For this review, take the finished solid that the model builds, in its own axes (mm). Face numbers are marked on the shaded views. Round coordinates to 2 decimals unless told otherwise and drop trailing zeros. Write each loop counter-clockwise with the first axis right and the second up, starting at its lowest first coordinate (ties: lowest second). Pieces come first, ordered by that corner, then holes. Notation, with made-up numbers: (76.25, 85.25) -> (128.25, 85.25) arc R14 cw to (128.25, 91.25) -> close; hole circle Ø3 at (-21, 77). An arc over 180 degrees is marked (long way). Answer in a Markdown table with one row per item.
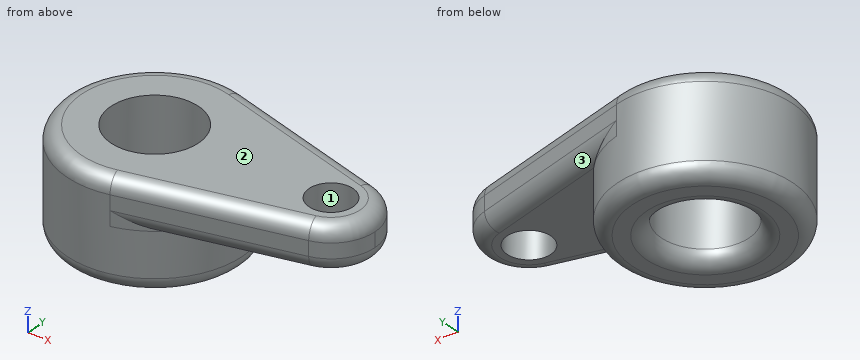
from build123d import *
from build123d import SkipClean  # not in build123d's __all__

# Parameters (mm, degrees)
F0_R         = 15
F0_R_2       = 7.5
F1_DEPTH     = 15
F2_DEPTH     = 20
F3_R         = 5
F4_T1_DEPTH  = 58.0947501931
F4_T3_DEPTH  = 58.0947501931
F4_T8_DEPTH  = 79.3447501931
F4_S9_R      = 30
F4_T10_DEPTH = 43
F4_T12_ANGLE = 151.0449756281
F4_T14_ANGLE = 151.0449756281
F4_T18_DEPTH = 79.3447501931
F4_S19_R     = 30
F4_T20_DEPTH = 43
F4_T22_ANGLE = 208.9550243719


# Not quite as in the source:
# - a fillet or chamfer that OpenCascade refuses, or shapes differently, is made with other operations: its cross-section is extruded or revolved along the edge and cut away or added


with BuildPart() as f1:
    # F0 (on Top) → F1 (new body)
    with BuildSketch(Plane.XY):
        with BuildLine():
            ThreePointArc((7.5, -29.0473750966), (23.7170824513, -18.3711730709), (30, 0))
            ThreePointArc((30, 0), (23.7170824513, 18.3711730709), (7.5, 29.0473750966))
            ThreePointArc((7.5, 29.0473750966), (-30, 0), (7.5, -29.0473750966))
        make_face()
        Circle(F0_R, mode=Mode.SUBTRACT)
        with BuildLine():
            ThreePointArc((7.5, 29.0473750966), (23.7170824513, 18.3711730709), (30, 0))
            ThreePointArc((30, 0), (23.7170824513, -18.3711730709), (7.5, -29.0473750966))
            Line((7.5, -29.0473750966), (63.75, -14.5236875483))
            ThreePointArc((63.75, -14.5236875483), (45, 0), (63.75, 14.5236875483))
            Line((63.75, 14.5236875483), (7.5, 29.0473750966))
        make_face()
        with BuildLine():
            ThreePointArc((75, 0), (71.8585412256, 9.1855865354), (63.75, 14.5236875483))
            ThreePointArc((63.75, 14.5236875483), (45, 0), (63.75, -14.5236875483))
            ThreePointArc((63.75, -14.5236875483), (71.8585412256, -9.1855865354), (75, 0))
        make_face()
        with Locations((60, 0)):
            Circle(F0_R_2, mode=Mode.SUBTRACT)
    extrude(amount=F1_DEPTH)

    # F0 (on Top) → F2 (join)
    with BuildSketch(Plane.XY):
        with BuildLine():
            ThreePointArc((7.5, -29.0473750966), (23.7170824513, -18.3711730709), (30, 0))
            ThreePointArc((30, 0), (23.7170824513, 18.3711730709), (7.5, 29.0473750966))
            ThreePointArc((7.5, 29.0473750966), (-30, 0), (7.5, -29.0473750966))
        make_face()
        Circle(F0_R, mode=Mode.SUBTRACT)
    with SkipClean():  # cleaning this boolean's faces spoils the solid; the shape is the same uncleaned
        extrude(amount=-F2_DEPTH)

    # F3
    f3_edges = [f1.edges().sort_by_distance(p)[0] for p in [
        (-7.5, 29.047375, -20),
        (-15, 0, -20),
    ]]
    fillet(f3_edges, radius=F3_R)

    # F4: fillet of radius 5 on 11 edges, made by hand

    # F4_s2 → F4_t1 (cut)
    with BuildSketch(Plane(origin=(0, 0, 0), x_dir=(0, 0, 1), z_dir=(0.9682458366, 0.25, 0))):
        with BuildLine():
            ThreePointArc((10, 30), (13.5355339059, 28.5355339059), (15, 25))
            Line((15, 25), (15, 30))
            Line((15, 30), (10, 30))
        make_face()
    extrude(amount=F4_T1_DEPTH, mode=Mode.SUBTRACT)

    # F4_s4 → F4_t3 (cut)
    with BuildSketch(Plane(origin=(56.25, -14.5236875483, 0), x_dir=(0, 0, 1), z_dir=(-0.9682458366, 0.25, 0))):
        with BuildLine():
            ThreePointArc((10, 30), (13.5355339059, 28.5355339059), (15, 25))
            Line((15, 25), (15, 30))
            Line((15, 30), (10, 30))
        make_face()
    extrude(amount=F4_T3_DEPTH, mode=Mode.SUBTRACT)


with BuildPart() as f4_tool6:
    # F4_s7 → F4_t8 (new body)
    with BuildSketch(Plane(origin=(-20.5752240267, -5.3125, 0), x_dir=(0, 0, 1), z_dir=(0.9682458366, 0.25, 0))):
        with BuildLine():
            ThreePointArc((0, 25), (1.4644660941, 28.5355339059), (5, 30))
            Line((5, 30), (0, 30))
            Line((0, 30), (0, 25))
        make_face()
    extrude(amount=F4_T8_DEPTH)

    # F4_s9 → F4_t10 (cut, symmetric)
    with BuildSketch(Plane.XY.offset(2.5)):
        Circle(F4_S9_R)
    extrude(amount=F4_T10_DEPTH, both=True, mode=Mode.SUBTRACT)


with BuildPart() as f1_1:
    add(f1.part, clean=False)

    # F4_t5: cut F4_tool6
    add(f4_tool6.part, mode=Mode.SUBTRACT)

    # F4_s11 → F4_t12 (revolve, cut)
    with BuildSketch(Plane(origin=(56.25, 14.5236875483, 0), x_dir=(0, 0, 1), z_dir=(-0.9682458366, -0.25, 0))):
        with BuildLine():
            ThreePointArc((0, -25), (1.4644660941, -28.5355339059), (5, -30))
            Line((5, -30), (0, -30))
            Line((0, -30), (0, -25))
        make_face()
    revolve(axis=Axis((60, 0, 0), (0, 0, 1)), revolution_arc=F4_T12_ANGLE, mode=Mode.SUBTRACT)

    # F4_s13 → F4_t14 (revolve, cut)
    with BuildSketch(Plane(origin=(56.25, 14.5236875483, 0), x_dir=(0, 0, 1), z_dir=(-0.9682458366, -0.25, 0))):
        with BuildLine():
            ThreePointArc((15, -25), (13.5355339059, -28.5355339059), (10, -30))
            Line((10, -30), (15, -30))
            Line((15, -30), (15, -25))
        make_face()
    revolve(axis=Axis((60, 0, 15), (0, 0, 1)), revolution_arc=F4_T14_ANGLE, mode=Mode.SUBTRACT)


with BuildPart() as f4_tool16:
    # F4_s17 → F4_t18 (new body)
    with BuildSketch(Plane(origin=(56.25, -14.5236875483, 0), x_dir=(0, 0, 1), z_dir=(-0.9682458366, 0.25, 0))):
        with BuildLine():
            ThreePointArc((0, 25), (1.4644660941, 28.5355339059), (5, 30))
            Line((5, 30), (0, 30))
            Line((0, 30), (0, 25))
        make_face()
    extrude(amount=F4_T18_DEPTH)

    # F4_s19 → F4_t20 (cut, symmetric)
    with BuildSketch(Plane.XY.offset(2.5)):
        Circle(F4_S19_R)
    extrude(amount=F4_T20_DEPTH, both=True, mode=Mode.SUBTRACT)


with BuildPart() as f1_2:
    add(f1_1.part, clean=False)

    # F4_t15: cut F4_tool16
    add(f4_tool16.part, mode=Mode.SUBTRACT)

    # F4_s21 → F4_t22 (revolve, cut)
    with BuildSketch(Plane(origin=(0, 0, 0), x_dir=(0, 0, 1), z_dir=(0.9682458366, -0.25, 0))):
        with BuildLine():
            ThreePointArc((10, -30), (13.5355339059, -28.5355339059), (15, -25))
            Line((15, -25), (15, -30))
            Line((15, -30), (10, -30))
        make_face()
    revolve(axis=Axis((0, 0, 15), (0, 0, 1)), revolution_arc=F4_T22_ANGLE, mode=Mode.SUBTRACT)


solid = f1_2.part
1) Mouldability with a two-part tool opening along Y and no side actions: class the marked faces 1, 2 and 3 as pulls with the +Y half, pulls with the -Y half, needs draft (parallel to the pull), parting line crosses it, or undercut.
Solved:
| item | result |
|---|---|
| face 1 | undercut |
| face 2 | needs draft |
| face 3 | pulls with the +Y half |
2) Consider section A-A on z = -5.5. State the section outline as (x, y) points, then the cut area to 3 significant figures.
Solved:
| item | result |
|---|---|
| outline | circle Ø60 at (0, 0); hole circle Ø30 at (0, 0) |
| area | 2,120 mm² |
3) Consider section B-B on y = -6. State how many separate pieces and enclosed holes the cut face has, then the cut area to 3 significant figures.
Solved:
| item | result |
|---|---|
| separate pieces | 3 |
| enclosed holes | 0 |
| area | 1,590 mm² |
4) For line 1 (Y direction, x = 0, z = -6); line 2 (Z direction, x = 45.5, y = -8.5); line 3 (Y direction, x = 60, z = 12.25), list the stretches that pass through material, from the lowest coordinate up. Write a range as [from, to].
Solved:
| item | result |
|---|---|
| line 1 | [-30, -15], [15, 30] |
| line 2 | [0, 15] |
| line 3 | [-14.94, -7.5], [7.5, 14.94] |
5) Clearance check with flat-ended pins moving along their axes: pin 1 Ø9 at (x, y) = (60, 0) entering from -Z; pin 2 Ø1.5 at (y, z) = (23, 3.5) entering from -X; pin 3 Ø1.5 at (x, y) = (29.5, 12) entering from -Z; pin 4 Ø1.5 at (x, z) = (36.5, 3) entering from +Y. State where each tip first meets the part, or that it passes through.
Solved:
| item | result |
|---|---|
| pin 1 | through |
| pin 2 | x = -20.12 |
| pin 3 | z = 0 |
| pin 4 | y = 21.47 |
